Check sheet for the modelled part. Datum: model origin and axes. Units: mm. Face numbers are marked on the shaded views. A direction names the side the tool comes from. Round coordinates to 2 decimals unless told otherwise and drop trailing zeros. Order: outer loops, then holes, each group sorted by start corner. A loop starts at its lowest first (then second) coordinate and runs counter-clockwise, first axis right, second up.
(1) Thickness scan on probe 1 along X at (y, z) = (-1, 9); probe 2 along Z at (x, y) = (16, -12); probe 3 along Y at (x, z) = (11.5, 18). Record the ranges inside material, lowest first.
(2) Tool access check on the marked faces 1, 2 and 3. Record the directions out of +Z, -Z, +X, -X, +Y, -Y that give a thin tool (end or side, any length) a straight path to the whole face; none if there is none.
(3) Sectioned sample at D-D, the plane y = -25. Enter the section's corners in (x, z).
(4) Depth check by flat-ended pin: pin 1 (5 mm diameter, centred on x = 4, z = 27.5, fed in from +Y); pin 2 (4 mm diameter, centred on y = -18, z = 27.5, fed in from +X); pin 3 (3.5 mm diameter, centred on y = -5, z = 16, fed in from -X). Enter the tip coordinate at first touch or a pass-through.
(5) Sectioned sample at C-C, the plane x = 19.5. Enter the section's corners in (y, z), and give its area (3 significant figures).
(6) Sectioned sample at B-B, the plane y = -15. Enter the section's corners in (x, z).
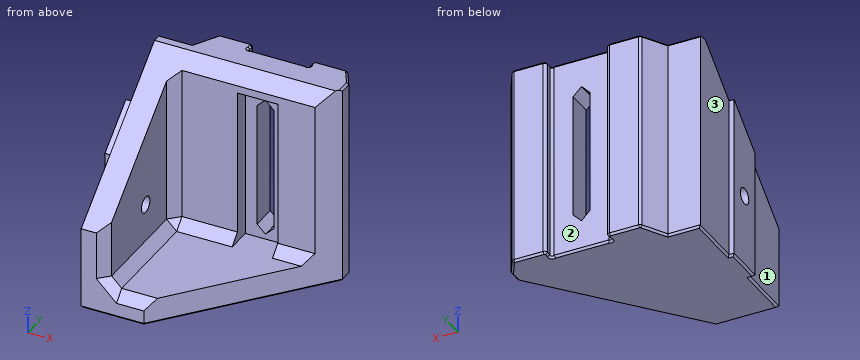
```python
from build123d import *

# Parameters (mm, degrees)
BOSS_EXTRUDE1_DEPTH = 40
CUT_EXTRUDE1_DEPTH  = 35
CUT_EXTRUDE2_DEPTH  = 38.586751346
BOSS_EXTRUDE2_DEPTH = 1
SKETCH5_R           = 1.6
CUT_EXTRUDE3_DEPTH  = 39.586751346
CHAMFER2_SIZE       = 1.3
CHAMFER2_SIZE2      = 1.671247785
FILLET1_R           = 0.6
CUT_EXTRUDE4_DEPTH  = 34
SKETCH7_W           = 8
SKETCH7_H           = 31
CUT_EXTRUDE5_DEPTH  = 3
CHAMFER3_SIZE       = 2
CHAMFER4_SIZE       = 0.4


with BuildPart() as part:
    # Sketch1 → Boss-Extrude1 (new body)
    with BuildSketch(Plane.XY):
        with BuildLine():
            Line((0, 0), (0, -30))
            Line((0, -30), (12.413762411, -30))
            Line((12.413762411, -30), (37.586751346, 0))
            Line((37.586751346, 0), (34.7, 5))
            Line((34.7, 5), (28, 5))
            Line((28, 5), (28, 3.565685425))
            ThreePointArc((28, 3.565685425), (28, 3), (27.434314575, 3))
            Line((27.434314575, 3), (16.573996535, 3))
            ThreePointArc((16.573996535, 3), (16.008373082, 2.991626918), (16, 3.557250372))
            Line((16, 3.557250372), (16, 5))
            Line((16, 5), (9.3, 5))
            Line((9.3, 5), (6.413248654, 0))
            Line((6.413248654, 0), (0, 0))
        make_face()
    extrude(amount=BOSS_EXTRUDE1_DEPTH)

    # Sketch2 → Cut-Extrude1 (cut)
    with BuildSketch(Plane.XY.offset(40)):
        Polygon((5, -5), (5, -30), (12.413762411, -30), (33.39125319, -5), align=None)
    extrude(amount=-CUT_EXTRUDE1_DEPTH, mode=Mode.SUBTRACT)

    # Sketch3 → Cut-Extrude2 (cut, through all)
    with BuildSketch(Plane.ZY):
        Polygon((40, -30), (40, -2), (16.505210327, -30), align=None)
    extrude(amount=-CUT_EXTRUDE2_DEPTH, mode=Mode.SUBTRACT)

    # Sketch4 → Boss-Extrude2 (add)
    with BuildSketch(Plane.ZY):
        Polygon((0, -11), (0, -19), (25.73530627, -19), (32.448103319, -11), align=None)
    extrude(amount=BOSS_EXTRUDE2_DEPTH)

    # Sketch5 → Cut-Extrude3 (cut, through all)
    with BuildSketch(Plane.ZY.offset(1)):
        with Locations((14.545852397, -15)):
            Circle(SKETCH5_R)
    extrude(amount=-CUT_EXTRUDE3_DEPTH, mode=Mode.SUBTRACT)

    # Chamfer2
    chamfer2_edges = [part.edges().sort_by_distance(p)[0] for p in [
        (37.586751346, 0, 20),
    ]]
    chamfer2_side = [part.faces().sort_by_distance(p)[0] for p in [
        (25.000256878, -15, 0.559792763),
    ]]
    chamfer(chamfer2_edges, length=CHAMFER2_SIZE, length2=CHAMFER2_SIZE2, reference=chamfer2_side[0])

    # Fillet1
    fillet1_edges = [part.edges().sort_by_distance(p)[0] for p in [
        (9.3, 5, 20),
        (16, 5, 20),
        (28, 5, 20),
        (34.7, 5, 20),
    ]]
    fillet(fillet1_edges, radius=FILLET1_R)

    # Sketch6 → Cut-Extrude4 (cut, through all)
    with BuildSketch(Plane(origin=(0, 3, 0), x_dir=(1, 0, 0), z_dir=(0, 1, 0))):
        Polygon((22.004155555, -6), (20.354155555, -7.65), (20.354155555, -32.35), (22.004155555, -34), (23.654155555, -32.35), (23.654155555, -7.65), align=None)
    extrude(amount=-CUT_EXTRUDE4_DEPTH, mode=Mode.SUBTRACT)

    # Sketch7 → Cut-Extrude5 (cut)
    with BuildSketch(Plane.XZ.offset(5)):
        with Locations((22.004155555, 20.5)):
            Rectangle(SKETCH7_W, SKETCH7_H)
    extrude(amount=-CUT_EXTRUDE5_DEPTH, mode=Mode.SUBTRACT)

    # Chamfer3
    chamfer3_edges = [part.edges().sort_by_distance(p)[0] for p in [
        (29.697704373, -5, 5),
        (5, -5, 21.241350553),
        (8.706881205, -30, 5),
        (5, -30, 10.752605164),
        (11.502077778, -5, 5),
        (5, -17.5, 5),
    ]]
    chamfer(chamfer3_edges, length=CHAMFER3_SIZE)

    # Chamfer4
    chamfer4_edges = [part.edges().sort_by_distance(p)[0] for p in [
        (31.476794919, 5, 0),
        (31.476794919, 5, 40),
        (7.770021787, 2.35, 0),
        (12.523205081, 5, 0),
        (28, 3.982842712, 0),
        (28.175735931, 4.824264069, 0),
        (9.346410162, 4.919615242, 0),
        (15.824264069, 4.824264069, 0),
        (34.653589838, 4.919615242, 0),
        (28, 3.982842712, 40),
        (12.523205081, 5, 40),
        (7.770021787, 2.35, 40),
        (28.175735931, 4.824264069, 40),
        (9.346410162, 4.919615242, 40),
        (15.824264069, 4.824264069, 40),
        (34.653589838, 4.919615242, 40),
        (16, 3.978625186, 0),
        (16.008373082, 2.991626918, 0),
        (22.004155555, 3, 0),
        (28, 3, 0),
        (24.582444932, -15.497928888, 0),
        (6.206881205, -30, 0),
        (0, -5.5, 0),
        (3.206624327, 0, 0),
        (28, 3, 40),
        (22.004155555, 3, 40),
        (16.008373082, 2.991626918, 40),
        (16, 3.978625186, 40),
        (3.206624327, 0, 40),
        (0, -24.5, 0),
        (-0.5, -11, 0),
        (-0.5, -19, 0),
        (-1, -15, 0),
        (35.812166267, 3.073671519, 0),
        (35.812166267, 3.073671519, 40),
        (36.751127453, 0.225742631, 0),
        (36.751127453, 0.225742631, 40),
    ]]
    chamfer(chamfer4_edges, length=CHAMFER4_SIZE)


solid = part.part
```
Derived:
1. probe 1: x = 0 to 20.35, 23.65 to 36.75
1. probe 2: z = 0 to 5
1. probe 3: y = -5 to 5
2. face 1: +Z, -Z, -X, -Y
2. face 2: +Z, -Z, +Y
2. face 3: +Z, -Z, -X, +Y
3. outline: (0, 0.4) - (0.4, 0) - (16.09, 0) - (16.61, 0.4) - (16.61, 5) - (7, 5) - (5, 7) - (5, 20.7) - (0, 20.7) - close
4. pin 1: stops at y = 0.15
4. pin 2: stops at x = 5
4. pin 3: stops at x = 0
5. outline: (-21.55, 0.4) - (-20.93, 0) - (2.6, 0) - (3, 0.4) - (3, 39.6) - (2.6, 40) - (-2, 40) - (-5, 37.48) - (-5, 36) - (-2, 36) - (-2, 5) - (-21.55, 5) - close
5. area: 306 mm2
6. outline: (-1, 0.4) - (-0.6, 0) - (24.48, 0) - (25, 0.4) - (25, 5) - (7, 5) - (5, 7) - (5, 12.95) - (-1, 12.95) - close; (-1, 16.15) - (5, 16.15) - (5, 29.09) - (-1, 29.09) - close
